from build123d import *

# Parameters (mm, degrees)
BOSS_EXTRUDE1_DEPTH = 4
BOSS_EXTRUDE1_DRAFT = 1
SHELL1_T            = -0.5
SKETCH2_R           = 2
BOSS_EXTRUDE2_DEPTH = 5.5
BOSS_EXTRUDE2_TAPER = 1.5
CIRPATTERN1_COUNT   = 4


with BuildPart() as part:
    # Sketch1 → Boss-Extrude1 (with draft: the straight prism first)
    with BuildSketch(Plane(origin=(0, 0, 0), x_dir=(1, 0, 0), z_dir=(0, 1, 0))):
        with BuildLine():
            Line((-7.5, -4), (7.5, -4))
            ThreePointArc((7.5, -4), (8.207106781, -3.707106781), (8.5, -3))
            Line((8.5, -3), (8.5, 3))
            ThreePointArc((8.5, 3), (8.207106781, 3.707106781), (7.5, 4))
            Line((7.5, 4), (-7.5, 4))
            ThreePointArc((-7.5, 4), (-8.207106781, 3.707106781), (-8.5, 3))
            Line((-8.5, 3), (-8.5, -3))
            ThreePointArc((-8.5, -3), (-8.207106781, -3.707106781), (-7.5, -4))
        make_face()
    extrude(amount=-BOSS_EXTRUDE1_DEPTH)
    # Boss-Extrude1: the draft: its side faces are tilted about the plane it starts from
    boss_extrude1_sides = [part.faces().sort_by_distance(p)[0] for p in [
        (0, -2, 4),
        (8.207106781, -2, 3.707106781),
        (8.5, -2, 0),
        (8.207106781, -2, -3.707106781),
        (0, -2, -4),
        (-8.207106781, -2, -3.707106781),
        (-8.5, -2, 0),
        (-8.207106781, -2, 3.707106781),
    ]]
    draft(boss_extrude1_sides, Plane(origin=(0, 0, 0), x_dir=(1, 0, 0), z_dir=(0, 1, 0)), BOSS_EXTRUDE1_DRAFT)

    # Shell1
    shell1_openings = [part.faces().sort_by_distance(p)[0] for p in [
        (0, -4, 0),
    ]]
    offset(amount=SHELL1_T, openings=shell1_openings, kind=Kind.INTERSECTION)

    # Sketch2 → Boss-Extrude2 (add)
    with BuildSketch(Plane.XZ.offset(0.5)):
        Circle(SKETCH2_R)
    extrude(amount=BOSS_EXTRUDE2_DEPTH, taper=BOSS_EXTRUDE2_TAPER)

    # Rib1: read off the stored shape, not the designer's step
    # Rib1: loft between two sections, ruled curve by curve
    rib1_from = [
        Edge.make_line((1.982021382, -0.5, 0.267565397), (3, -0.5, 0.25)),
        Edge.make_line((1.982021382, -0.5, -0.267565397), (3, -0.5, -0.25)),
        Edge.make_line((3, -0.5, -0.25), (3, -0.5, 0.25)),
        Edge.make_line((1.982021382, -0.5, -0.267565397), (1.982021382, -0.5, 0.267565397)),
    ]
    rib1_to = [
        Edge.make_line((1.877498903, -4.5, 0.258832698), (2.38938588, -4.5, 0.25)),
        Edge.make_line((1.877498903, -4.5, -0.258832698), (2.38938588, -4.5, -0.25)),
        Edge.make_line((2.38938588, -4.5, -0.25), (2.38938588, -4.5, 0.25)),
        Edge.make_line((1.877498903, -4.5, -0.258832698), (1.877498903, -4.5, 0.258832698)),
    ]
    rib1 = Solid(Shell([*[Face.make_surface_from_curves(rib1_from[k], rib1_to[k]) for k in range(4)], Face(Wire(rib1_from)), Face(Wire(rib1_to))]))
    add(rib1)

    # CirPattern1: Rib1 ×4 about axis
    cirpattern1_axis = Axis((0, 0, 0), (0, 1, 0))
    for i in range(1, CIRPATTERN1_COUNT):
        add(rib1.rotate(cirpattern1_axis, i * 360 / CIRPATTERN1_COUNT))


solid = part.part
Check sheet for the modelled part. Datum: model origin and axes. Units: mm. A direction names the side the tool comes from. Give positions to 0.01 mm unless a question says otherwise; leave off trailing zeros. Loops run counter-clockwise (first coordinate to the right, second up) from the corner with the lowest first, then second, coordinate; pieces in that order, holes last. Notation, with made-up numbers: M 80,7.25 L 103,7.25 A29 ccw 103,41.25 Z; hole C -34,34.5 d6. An arc over 180 degrees is marked long. Use a Markdown table: item, result. Add a question column.
Q1. Mould release check, pull along Z, two halves, no side actions. Record for faces 1 (the conical face through (-8.24, -1.97, 3.72)), 2 (the conical face through (0.89, -3.29, -1.71)), 3 (the flat face through (0, -6, 0)): pulls with the +Z half, pulls with the -Z half, needs draft (parallel to the pull), parting line crosses it, or undercut.
Q2. Sectioned sample at B-B, the plane y = -2.5. Give the number of separate pieces and of enclosed holes in the cut face, then the cut area to 3 significant figures.
Q3. Tool access check on faces 4 (the conical face through (8.22, -1.97, 3.74)), 5 (the flat face through (-2, -0.5, -1)), 6 (the conical face through (-8.22, -1.97, -3.74)). Record the directions out of +Z, -Z, +X, -X, +Y, -Y that give a thin tool (end or side, any length) a straight path to the whole face; none if there is none.
Q4. Scan lines: line 1 along X through (y, z) = (-1, 1); line 2 along X through (y, z) = (-3, -1.25); line 3 along Y through (x, z) = (-1.5, -2.25). Record each from-to range of solid material in increasing order. Write a range as [from, to].
Q5. Sectioned sample at A-A, the plane x = -4.5. Record the cut outline in (y, z).
Q6. Go/stop test with flat-tipped pins: pin 1 (3 mm diameter, centred on y = -2, z = 3, fed in from +X); pin 2 (1 mm diameter, centred on x = 4, y = -5, fed in from +Z). Record where each tip stops, or that it passes through.
Q7. Sectioned sample at D-D, the plane y = -5.25. Record the cut outline in (x, z), then the cut area to 3 significant figures.
Verdict:
| question | item | result |
|---|---|---|
| 1 | face 1 | pulls with the +Z half |
| 1 | face 2 | undercut |
| 1 | face 3 | needs draft |
| 2 | separate pieces | 2 |
| 2 | enclosed holes | 1 |
| 2 | area | 37.0 mm^2 |
| 3 | face 4 | +Z, +X, +Y |
| 3 | face 5 | -Y |
| 3 | face 6 | -Z, -X, +Y |
| 4 | line 1 | [-8.52, -8.02], [-1.72, 1.72], [8.02, 8.52] |
| 4 | line 2 | [-8.55, -8.05], [-1.48, 1.48], [8.05, 8.55] |
| 4 | line 3 | [-0.5, 0] |
| 5 | outline | M -4,-4.07 L 0,-4 L 0,4 L -4,4.07 L -4,3.57 L -0.5,3.51 L -0.5,-3.51 L -4,-3.57 Z |
| 6 | pin 1 | x = 8.56 |
| 6 | pin 2 | through |
| 7 | outline | C 0,0 d3.75 |
| 7 | area | 11.1 mm^2 |
